Autodesk Inventor part; units mm, degrees
ref_plane "Arbeitsebene1" through (-4, 0, -46) normal (0, 1, 0) x (0, 0, 1)
ref_plane "YZ Plane" through (0, 0, 0) normal (1, 0, 0) x (0, 1, 0)
ref_plane "XZ Plane" through (0, 0, 0) normal (0, 1, 0) x (-1, 0, 0)
sketch "Skizze1" plane through (0, 0, 0) normal (0, 0, 1) x (1, 0, 0)
  line L0 (-9.8, 0) -> (9.8, 0)
  line L1 (0, -9.8) -> (0, 9.8)
  line L2 (-7, 7) -> (7, 7)
  line L3 (7, 7) -> (7, -7)
  line L4 (7, -7) -> (-7, -7)
  line L5 (-7, -7) -> (-7, 7)
  point P0 (0, 0)
  dimension "d0" = 14
  dimension "d1" = 14
extrude "Extrusion1" add sketch "Skizze1" along normal mid plane 92
sketch "Skizze2" plane through (-7, -7, 46) normal (0, -1, 0) x (1, 0, 0)
  line L0 (0, 0) -> (14, 0)
  line L1 (0, 0) -> (0, -92)
  line L2 (14, -92) -> (0, -92)
  line L3 (3, 0) -> (11, 0)
  line L4 (11, 0) -> (11, -12)
  line L5 (11, -12) -> (3, -12)
  line L6 (3, -12) -> (3, 0)
  line L7 (3, -92) -> (11, -92)
  line L8 (11, -92) -> (11, -84)
  line L9 (11, -84) -> (3, -84)
  line L10 (3, -84) -> (3, -92)
  point P0 (7, -46)
  dimension "d6" = 8
  dimension "d7" = 12
  dimension "d8" = 8
  dimension "d9" = 3
extrude "Extrusion2" cut sketch "Skizze2" against normal through all
sketch "Skizze3" plane through (-4, -7, 34) normal (0, 0, 1) x (1, 0, 0)
  line L0 (8, 0) -> (8, 14)
  line L1 (0, 0) -> (8, 0)
  line L2 (8, 0) -> (8, 8)
  line L3 (8, 8) -> (0, 8)
  line L4 (0, 8) -> (0, 0)
  point P0 (4, 7)
  dimension "d12" = 8
extrude "Extrusion3" cut sketch "Skizze3" against normal through all
sketch "Skizze4" plane through (-4, 7, 34) normal (0, 0, 1) x (1, 0, 0)
  line L0 (0, 0) -> (8, 0)
  line L1 (0, -6) -> (0, 0)
  point P0 (4, -7)
  point P1 (4, -4)
  dimension "d15" = 4
  dimension "d16" = 4
hole "Bohrung1" at (0, 3, 34) direction (0, 0, -1) diameter 2.459 depth 7 tip angle 118
sketch "Skizze5" plane through (7, 7, 46) normal (0, 1, 0) x (1, 0, 0)
  line L0 (-11, 84) -> (-3, 84)
  line L1 (-3, 84) -> (-3, 92)
  line L2 (-3, 92) -> (-11, 92)
  line L3 (-11, 92) -> (-11, 84)
  point P0 (-7, 46)
ref_plane "Arbeitsebene1" through (-4, 0, -46) normal (0, 1, 0) x (0, 0, 1)
extrude "Extrusion4" add sketch "Skizze5" against normal blind 6
sketch "Skizze6" plane through (-7, -7, 46) normal (-1, 0, 0) x (0, 0, 1)
  line L0 (0, 0) -> (-92, 0)
  line L1 (-84.5, 7) -> (-27.5, 7) construction
  line L2 (-84.5, 3.5) -> (-27.5, 3.5)
  line L3 (-27.5, 10.5) -> (-84.5, 10.5)
  arc A0 (-84.5, 10.5) -> (-84.5, 3.5) centre (-84.5, 7) ccw
  arc A1 (-27.5, 3.5) -> (-27.5, 10.5) centre (-27.5, 7) ccw
  line L4 (0, 14) -> (0, 0)
  point P0 (-92, 14)
  point P1 (-46, 7)
  point P2 (-56, 7)
  dimension "d26" = 64
  dimension "d27" = 7
  dimension "d28" = 92
  dimension "d30" = 7
  dimension "d40" = 24
extrude "Extrusion5" cut sketch "Skizze6" against normal blind 1.5
sketch "Skizze7" plane through (-7, 7, -46) normal (0, 1, 0) x (1, 0, 0)
  line L0 (11, -80) -> (11, -92)
  line L1 (14, -92) -> (11, -92)
  line L2 (14, -92) -> (14, 0)
  line L3 (7, -25) -> (7, -64.5) construction
  line L4 (3.5, -25) -> (3.5, -64.5)
  line L5 (10.5, -64.5) -> (10.5, -25)
  arc A0 (10.5, -25) -> (3.5, -25) centre (7, -25) ccw
  arc A1 (3.5, -64.5) -> (10.5, -64.5) centre (7, -64.5) ccw
  point P0 (7, -46)
  point P1 (7, -44.75)
  dimension "d33" = 7
  dimension "d34" = 7
  dimension "d36" = 46.5
  dimension "d41" = 24
extrude "Extrusion6" cut sketch "Skizze7" against normal blind 1.5
ref_plane "Arbeitsebene2" through (0, -7, 46) normal (1, 0, 0) x (0, 0, -1)
mirror "Spiegeln1" about plane through (0, -7, 46) normal (1, 0, 0) of "Extrusion5"
sketch "Skizze8" plane through (0, 0, -46) normal (0, 0, -1) x (-1, 0, 0)
  line L0 (-7, -7) -> (-4, -7)
  line L1 (-5.5, -7) -> (5.5, -7)
  line L2 (5.5, -7) -> (5.5, -6)
  line L3 (5.5, -6) -> (-5.5, -6)
  line L4 (-5.5, -6) -> (-5.5, -7)
  point P0 (0, 0)
  dimension "d42" = 11
  dimension "d43" = 1
extrude "Extrusion7" cut sketch "Skizze8" against normal through all
sketch "Skizze9" plane through (-7, -7, 46) normal (-1, 0, 0) x (0, 0, 1)
  line L0 (-58, 9) -> (-54, 9)
  line L1 (-54, 5) -> (-58, 5)
  line L2 (-61, 4.5) -> (-51, 4.5)
  line L3 (-51, 9.5) -> (-61, 9.5)
  line L4 (-71.5, 5) -> (-75.5, 5)
  line L5 (-75.5, 9) -> (-71.5, 9)
  line L6 (-78.5, 4.5) -> (-68.5, 4.5)
  line L7 (-68.5, 9.5) -> (-78.5, 9.5)
  line L8 (-40.5, 9) -> (-36.5, 9)
  line L9 (-36.5, 5) -> (-40.5, 5)
  line L10 (-43.5, 4.5) -> (-33.5, 4.5)
  line L11 (-33.5, 9.5) -> (-43.5, 9.5)
  arc A0 (-58, 9) -> (-58, 5) centre (-58, 7) ccw
  arc A1 (-54, 5) -> (-54, 9) centre (-54, 7) ccw
  arc A2 (-61, 9.5) -> (-61, 4.5) centre (-61, 7) ccw
  arc A3 (-51, 4.5) -> (-51, 9.5) centre (-51, 7) ccw
  arc A4 (-40.5, 9) -> (-40.5, 5) centre (-40.5, 7) ccw
  arc A5 (-36.5, 5) -> (-36.5, 9) centre (-36.5, 7) ccw
  arc A6 (-43.5, 9.5) -> (-43.5, 4.5) centre (-43.5, 7) ccw
  arc A7 (-33.5, 4.5) -> (-33.5, 9.5) centre (-33.5, 7) ccw
  arc A8 (-71.5, 5) -> (-71.5, 9) centre (-71.5, 7) ccw
  arc A9 (-75.5, 9) -> (-75.5, 5) centre (-75.5, 7) ccw
  arc A10 (-78.5, 9.5) -> (-78.5, 4.5) centre (-78.5, 7) ccw
  arc A11 (-68.5, 4.5) -> (-68.5, 9.5) centre (-68.5, 7) ccw
  point P0 (-46, 7)
extrude "Extrusion8" cut sketch "Skizze9" against normal through all contours L0 A1 L1 A0 | L4 A9 L5 A8 | L8 A5 L9 A4
sketch "Skizze10" plane through (-7, 7, -46) normal (0, 1, 0) x (1, 0, 0)
  line L0 (5, -38) -> (5, -34)
  line L1 (9, -34) -> (9, -38)
  line L2 (4.5, -31) -> (4.5, -41)
  line L3 (9.5, -41) -> (9.5, -31)
  line L4 (9, -51.5) -> (9, -55.5)
  line L5 (5, -55.5) -> (5, -51.5)
  line L6 (4.5, -48.5) -> (4.5, -58.5)
  line L7 (9.5, -58.5) -> (9.5, -48.5)
  arc A0 (9, -51.5) -> (5, -51.5) centre (7, -51.5) ccw
  arc A1 (5, -55.5) -> (9, -55.5) centre (7, -55.5) ccw
  arc A2 (9.5, -48.5) -> (4.5, -48.5) centre (7, -48.5) ccw
  arc A3 (4.5, -58.5) -> (9.5, -58.5) centre (7, -58.5) ccw
  arc A4 (5, -38) -> (9, -38) centre (7, -38) ccw
  arc A5 (9, -34) -> (5, -34) centre (7, -34) ccw
  arc A6 (9.5, -31) -> (4.5, -31) centre (7, -31) ccw
  arc A7 (4.5, -41) -> (9.5, -41) centre (7, -41) ccw
  point P0 (7, -46)
extrude "Extrusion9" cut sketch "Skizze10" against normal through all contours L0 A5 L1 A4 | L4 A1 L5 A0
sketch "Skizze11" plane through (7, -7, 46) normal (1, 0, 0) x (0, 0, -1)
  arc A0 (27.5, 10.5) -> (27.5, 3.5) centre (27.5, 7) ccw
  arc A1 (84.5, 3.5) -> (84.5, 10.5) centre (84.5, 7) ccw
  point P0 (46, 7)
hole "Bohrung2" at (7, 0, 18.5) at (7, 0, -38.5) direction (-1, 0, 0) diameter 1.567 depth 3 tip angle 118
sketch "Skizze12" plane through (-7, -7, 46) normal (-1, 0, 0) x (0, 0, 1)
  arc A0 (-27.5, 3.5) -> (-27.5, 10.5) centre (-27.5, 7) ccw
  arc A1 (-84.5, 10.5) -> (-84.5, 3.5) centre (-84.5, 7) ccw
  point P0 (-46, 7)
hole "Bohrung3" at (-7, 0, 18.5) at (-7, 0, -38.5) direction (1, 0, 0) diameter 1.567 depth 3 tip angle 118
sketch "Skizze13" plane through (-7, 7, -46) normal (0, 1, 0) x (1, 0, 0)
  arc A0 (3.5, -64.5) -> (10.5, -64.5) centre (7, -64.5) ccw
  arc A1 (10.5, -25) -> (3.5, -25) centre (7, -25) ccw
  point P0 (7, -46)
hole "Bohrung4" at (0, 7, -21) at (0, 7, 18.5) direction (0, -1, 0) diameter 1.567 end through all
sketch "Skizze14" plane through (-7, 7, -46) normal (0, 1, 0) x (1, 0, 0)
  line L0 (0, 0) -> (14, 0)
  line L1 (3, -80) -> (11, -80)
  line L2 (7, 0) -> (7, -11.2044)
  point P0 (7, -46)
  point P1 (7, -4)
  dimension "d71" = 4
hole "Bohrung5" at (0, 7, -42) direction (0, -1, 0) diameter 3.4 end through all countersink diameter 6.9 countersink angle 90
sketch "Skizze15" plane through (-4, 1, -46) normal (0, -1, 0) x (1, 0, 0)
  line L0 (9.5, 80) -> (9.5, 0)
  line L1 (9.5, 0) -> (-1.5, 0)
  line L2 (-1.5, 0) -> (-1.5, 80)
  line L3 (-1.5, 80) -> (9.5, 80)
  circle A0 centre (4, 70) radius 1.25
  circle A1 centre (4, 10) radius 1.25
  circle A2 centre (4, 10) radius 1.25
  point P0 (4, 46)
  point P1 (4, 70)
  point P2 (4, 10)
hole "Bohrung6" at (0, 1, 24) at (0, 1, -36) direction (0, 1, 0) diameter 1.567 depth 5 tip angle 118
properties part number "13_1087_008" material "PVC, hart"
The model under review builds one solid part; all positions refer to its coordinate system, in mm. A direction names the side the tool comes from. Round coordinates to 2 decimals unless told otherwise and drop trailing zeros. Loops run counter-clockwise (first coordinate to the right, second up) from the corner with the lowest first, then second, coordinate; pieces in that order, holes last. Notation, with made-up numbers: (32, -0.75) - (79, -0.75) arc R12 ccw to (79, 17.25) - close; hole circle Ø6 at (25.5, 45). An arc over 180 degrees is marked (long way). Write each question's results on one line, items separated by ' | '. Start each with the question number.
Q1. Wall thickness on line 1 along Z through (x, y) = (4.3, 0); line 2 along X through (y, z) = (-5, -9.5); line 3 along X through (y, z) = (3.85, -36): over which ranges is each line inside the solid? List them lowest first. Write a range as [from, to].
Q2. Draft analysis for pull direction Y (two halves, no side actions). For faces 1 (the cylindrical face through (0.3, 3.218, 19.224)), 2 (the flat face through (5, -2, -27)), 3 (the conical face through (-0.693, 5.359, -40.329)), state which applies: pulls with the +Y half, pulls with the -Y half, needs draft (parallel to the pull), parting line crosses it, or undercut.
Q3. Insertion check: P1, Ø2.5, axis at x = -1.5, z = -37, coming from the -Y side; P2, Ø2, axis at x = 0, z = -42, coming from the -Y side; P3, Ø1, axis at x = -3, z = -26, coming from the -Y side. Each pin has a flat end and moves straight along its axis. Give the tip position at first contact, or say it passes through.
Q4. Take a section at A-A on z = 37. Give the boundary of the cut face in (x, y).
Q5. Take a section at D-D on z = -17. Give the boundary of the cut face in (x, y), plus the area to 3 significant figures.
Q6. Take a section at B-B on z = -27.5. Give the boundary of the cut face in (x, y).
Q7. Take a section at C-C on y = 0. Give the number of separate pieces and of enclosed holes in the cut face, plus the area to 3 significant figures.
Q8. Tool access review of faces 4 (the cylindrical face through (-0.53, 3.535, -35.423)), 5 (the flat face through (-5, -6, -1)), 6 (the cylindrical face through (6, 0, -42)), 7 (the cylindrical face through (-0.369, 1.827, 30.451)): name each direction out of +Z, -Z, +X, -X, +Y, -Y from which nothing blocks a thin tool from reaching the whole face with its end or side.
Data:
1) line 1: z = [-46, -39.28], [-37.72, -31.5], [-23.5, -14], [-6, 3.5], [11.5, 17.72], [19.28, 46] | line 2: x = [-7, -4], [4, 7] | line 3: x = [-7, -0.78], [0.78, 7]
2) face 1: needs draft | face 2: undercut | face 3: pulls with the +Y half
3) P1: stops at y = 1 | P2: passes through | P3: stops at y = 2
4) outline: (-7, -7) - (-5.5, -7) - (-5.5, -6) - (-4, -6) - (-4, 7) - (-7, 7) - close; (4, -6) - (5.5, -6) - (5.5, -7) - (7, -7) - (7, 7) - (4, 7) - close
5) outline: (-7, -7) - (-5.5, -7) - (-5.5, -6) - (-4, -6) - (-4, 1) - (4, 1) - (4, -6) - (5.5, -6) - (5.5, -7) - (7, -7) - (7, -3.5) - (5.5, -3.5) - (5.5, 3.5) - (7, 3.5) - (7, 7) - (3.5, 7) - (3.5, 5.5) - (-3.5, 5.5) - (-3.5, 7) - (-7, 7) - (-7, 3.5) - (-5.5, 3.5) - (-5.5, -3.5) - (-7, -3.5) - close | area: 97.5 mm²
6) outline: (-7, -7) - (-5.5, -7) - (-5.5, -6) - (-4, -6) - (-4, -2) - (-5.5, -2) - (-5.5, -3.5) - (-7, -3.5) - close; (-7, 3.5) - (-5.5, 3.5) - (-5.5, 2) - (5.5, 2) - (5.5, 3.5) - (7, 3.5) - (7, 7) - (-7, 7) - close; (4, -6) - (5.5, -6) - (5.5, -7) - (7, -7) - (7, -3.5) - (5.5, -3.5) - (5.5, -2) - (4, -2) - close
7) separate pieces: 12 | enclosed holes: 0 | area: 279 mm²
8) face 4: -Y | face 5: +Z, -Z, -Y | face 6: +X | face 7: +Z
